Can you work these out from the model? Positions are in its coordinate system, mm. Round coordinates to 2 decimals unless told otherwise and drop trailing zeros. Loops run counter-clockwise (first coordinate to the right, second up) from the corner with the lowest first, then second, coordinate; pieces in that order, holes last. Notation, with made-up numbers: (-33, -19) -> (24, -19) arc R19 ccw to (24, -12) -> close; hole circle Ø1 at (68.25, -26.5). An arc over 180 degrees is marked (long way). Use a Markdown table: item, result.
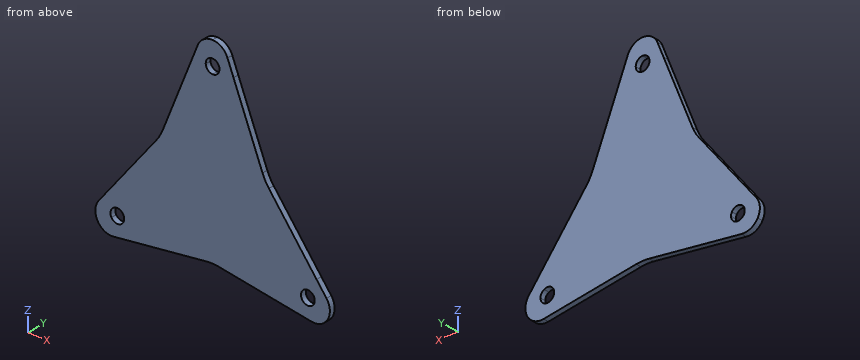
from build123d import *

# Parameters (mm, degrees)
F1_DEPTH = 6
F2_R     = 50
F3_R     = 50
F4_R     = 50


with BuildPart() as f1:
    # F0 (on Front) → F1 (new body)
    with BuildSketch(Plane.XZ):
        with BuildLine():
            ThreePointArc((107.4682422482, -53.390794226), (110.6754015758, -46.378394604), (113.4255666495, -39.1744920866))
            Line((113.4255666495, -39.1744920866), (57.0742879696, 32.9518555231))
            Line((57.0742879696, 32.9518555231), (0, 0))
            Line((0, 0), (97.4278579257, -56.25))
            ThreePointArc((97.4278579257, -56.25), (101.8689343878, -52.7867749652), (107.4682422482, -53.390794226))
        make_face()
        with BuildLine():
            Line((110.4182389825, -63.75), (125.5736835487, -72.5))
            ThreePointArc((125.5736835487, -72.5), (127.8756098621, -62.5292617095), (124.2084271706, -52.9759241818))
            Line((124.2084271706, -52.9759241818), (113.4255666495, -39.1744920866))
            ThreePointArc((113.4255666495, -39.1744920866), (110.6754015758, -46.378394604), (107.4682422482, -53.390794226))
            ThreePointArc((107.4682422482, -53.390794226), (110.3588449649, -56.1489581575), (111.4230484541, -60))
            ThreePointArc((111.4230484541, -60), (111.1674921513, -61.9411428383), (110.4182389825, -63.75))
        make_face()
        with BuildLine():
            ThreePointArc((90.6388886521, -78.6421761138), (95.5025687017, -72.6585120367), (99.9719052521, -66.374830774))
            ThreePointArc((99.9719052521, -66.374830774), (96.6491552976, -61.8276975537), (97.4278579257, -56.25))
            Line((97.4278579257, -56.25), (0, 0))
            Line((0, 0), (0, -65.9037110461))
            Line((0, -65.9037110461), (90.6388886521, -78.6421761138))
        make_face()
        with BuildLine():
            Line((-90.6388886521, -78.6421761138), (0, -65.9037110461))
            Line((0, -65.9037110461), (0, 0))
            Line((0, 0), (-97.4278579257, -56.25))
            ThreePointArc((-97.4278579257, -56.25), (-96.678604757, -58.0588571617), (-96.4230484541, -60))
            ThreePointArc((-96.4230484541, -60), (-97.3700501322, -63.6480423507), (-99.9719052521, -66.374830774))
            ThreePointArc((-99.9719052521, -66.374830774), (-95.5025687017, -72.6585120367), (-90.6388886521, -78.6421761138))
        make_face()
        with BuildLine():
            Line((0, 0), (-57.0742879696, 32.9518555231))
            Line((-57.0742879696, 32.9518555231), (-113.4255666495, -39.1744920866))
            ThreePointArc((-113.4255666495, -39.1744920866), (-110.6754015758, -46.378394604), (-107.4682422482, -53.390794226))
            ThreePointArc((-107.4682422482, -53.390794226), (-101.8689343878, -52.7867749652), (-97.4278579257, -56.25))
            Line((-97.4278579257, -56.25), (0, 0))
        make_face()
        with BuildLine():
            ThreePointArc((-124.2084271706, -52.9759241818), (-127.8756098621, -62.5292617095), (-125.5736835487, -72.5))
            Line((-125.5736835487, -72.5), (-110.4182389825, -63.75))
            ThreePointArc((-110.4182389825, -63.75), (-111.1362734889, -57.9458859336), (-107.4682422482, -53.390794226))
            ThreePointArc((-107.4682422482, -53.390794226), (-110.6754015758, -46.378394604), (-113.4255666495, -39.1744920866))
            Line((-113.4255666495, -39.1744920866), (-124.2084271706, -52.9759241818))
        make_face()
        with BuildLine():
            Line((-110.4182389825, -63.75), (-125.5736835487, -72.5))
            ThreePointArc((-125.5736835487, -72.5), (-118.0897340513, -79.4788958102), (-107.9827097157, -81.079691203))
            Line((-107.9827097157, -81.079691203), (-90.6388886521, -78.6421761138))
            ThreePointArc((-90.6388886521, -78.6421761138), (-95.5025687017, -72.6585120367), (-99.9719052521, -66.374830774))
            ThreePointArc((-99.9719052521, -66.374830774), (-105.7507460078, -67.2738931565), (-110.4182389825, -63.75))
        make_face()
        with BuildLine():
            ThreePointArc((0, 112.5), (-5.2197790902, 114.6144725189), (-7.4963369961, 119.765625))
            ThreePointArc((-7.4963369961, 119.765625), (-15.1728328741, 119.0369066406), (-22.7866779974, 117.8166682004))
            Line((-22.7866779974, 117.8166682004), (-57.0742879696, 32.9518555231))
            Line((-57.0742879696, 32.9518555231), (0, 0))
            Line((0, 0), (0, 112.5))
        make_face()
        with BuildLine():
            Line((0, 127.5), (0, 145))
            ThreePointArc((0, 145), (-9.7858758107, 142.0081575197), (-16.2257174549, 134.0556153848))
            Line((-16.2257174549, 134.0556153848), (-22.7866779974, 117.8166682004))
            ThreePointArc((-22.7866779974, 117.8166682004), (-15.1728328741, 119.0369066406), (-7.4963369961, 119.765625))
            ThreePointArc((-7.4963369961, 119.765625), (-5.3855274811, 125.2197790902), (0, 127.5))
        make_face()
        with BuildLine():
            ThreePointArc((16.2257174549, 134.0556153848), (9.7858758107, 142.0081575197), (0, 145))
            Line((0, 145), (0, 127.5))
            ThreePointArc((0, 127.5), (5.3033008589, 125.3033008589), (7.5, 120))
            ThreePointArc((7.5, 120), (7.4990841931, 119.8827981888), (7.4963369961, 119.765625))
            ThreePointArc((7.4963369961, 119.765625), (15.1728328741, 119.0369066406), (22.7866779974, 117.8166682004))
            Line((22.7866779974, 117.8166682004), (16.2257174549, 134.0556153848))
        make_face()
        with BuildLine():
            ThreePointArc((107.9827097157, -81.079691203), (118.0897340513, -79.4788958102), (125.5736835487, -72.5))
            Line((125.5736835487, -72.5), (110.4182389825, -63.75))
            ThreePointArc((110.4182389825, -63.75), (105.7507460078, -67.2738931565), (99.9719052521, -66.374830774))
            ThreePointArc((99.9719052521, -66.374830774), (95.5025687017, -72.6585120367), (90.6388886521, -78.6421761138))
            Line((90.6388886521, -78.6421761138), (107.9827097157, -81.079691203))
        make_face()
        with BuildLine():
            Line((57.0742879696, 32.9518555231), (22.7866779974, 117.8166682004))
            ThreePointArc((22.7866779974, 117.8166682004), (15.1728328741, 119.0369066406), (7.4963369961, 119.765625))
            ThreePointArc((7.4963369961, 119.765625), (5.2197790902, 114.6144725189), (0, 112.5))
            Line((0, 112.5), (0, 0))
            Line((0, 0), (57.0742879696, 32.9518555231))
        make_face()
    extrude(amount=F1_DEPTH)

    # F2
    f2_edges = [f1.edges().sort_by_distance(p)[0] for p in [
        (-57.074288, -3, 32.951856),
    ]]
    fillet(f2_edges, radius=F2_R)

    # F3
    f3_edges = [f1.edges().sort_by_distance(p)[0] for p in [
        (0, -3, -65.903711),
    ]]
    fillet(f3_edges, radius=F3_R)

    # F4
    f4_edges = [f1.edges().sort_by_distance(p)[0] for p in [
        (57.074288, -3, 32.951856),
    ]]
    fillet(f4_edges, radius=F4_R)


solid = f1.part
1. I want a section at C-C (z = 85). Please give me the cut outline in (x, y).
Answer sheet:
| item | result |
|---|---|
| outline | (-36.05, -6) -> (36.05, -6) -> (36.05, 0) -> (-36.05, 0) -> close |
2. Will these pins go through, and if not, where does the flat tip stop? pin 1 Ø1 at (y, z) = (-5.5, 34) entering from +X; pin 2 Ø1.5 at (x, y) = (-7, -3.5) entering from +Z; pin 3 Ø3 at (x, y) = (-15.5, -5) entering from +Z.
Answer sheet:
| item | result |
|---|---|
| pin 1 | stops at x = 57.33 |
| pin 2 | stops at z = 143.85 |
| pin 3 | stops at z = 138 |
3. I want a section at B-B (x = 102.5). Please give me the cut outline in (y, z).
Answer sheet:
| item | result |
|---|---|
| outline | (-6, -80.31) -> (0, -80.31) -> (0, -67.36) -> (-6, -67.36) -> close; (-6, -52.64) -> (0, -52.64) -> (0, -25.19) -> (-6, -25.19) -> close |
4. I need wall thicknesses on line 1 (Z direction, x = 4, y = -1.25); line 2 (Z direction, x = 80.5, y = -2.75); line 3 (X direction, y = -3.2, z = 118.5). Which ranges of each line are inside material? Lowest first, please.
Answer sheet:
| item | result |
|---|---|
| line 1 | z = -66.56 to 113.66, 126.34 to 144.54 |
| line 2 | z = -77.22 to 2.97 |
| line 3 | x = -22.51 to -7.35, 7.35 to 22.51 |
5. I want a section at D-D (x = 19.5). Please give me the cut outline in (y, z), plus the area to 3 significant figures.
Answer sheet:
| item | result |
|---|---|
| outline | (-6, -68.64) -> (0, -68.64) -> (0, 125.95) -> (-6, 125.95) -> close |
| area | 1,170 mm² |
6. I want a section at A-A (y = -4.5). Please give me the cut outline in (x, z), plus the area to 3 significant figures.
Answer sheet:
| item | result |
|---|---|
| outline | (-124.21, -52.98) arc R17.5 ccw to (-107.98, -81.08) -> (-6.96, -66.88) arc R50 cw to (6.96, -66.88) -> (107.98, -81.08) arc R17.5 ccw to (124.21, -52.98) -> (61.4, 27.41) arc R50 cw to (54.44, 39.47) -> (16.23, 134.06) arc R17.5 ccw to (-16.23, 134.06) -> (-54.44, 39.47) arc R50 cw to (-61.4, 27.41) -> close; hole circle Ø15 at (-103.92, -60); hole circle Ø15 at (0, 120); hole circle Ø15 at (103.92, -60) |
| area | 28,100 mm² |
